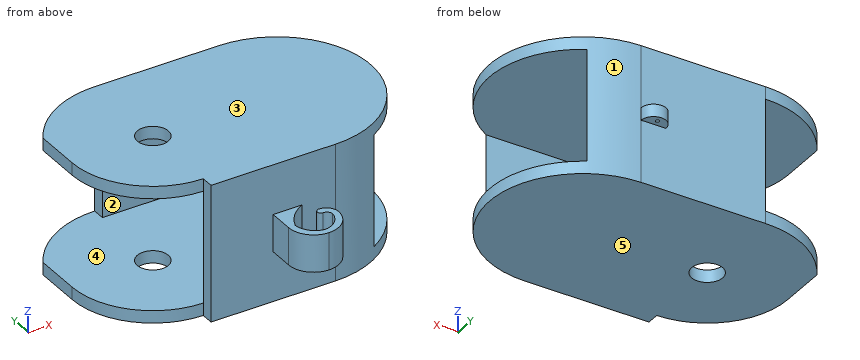
from build123d import *

# Parameters (mm, degrees)
SKETCH1_W           = 31.75
SKETCH1_H           = 19.05
BOSS_EXTRUDE1_DEPTH = 19.05
SKETCH2_R           = 1.5875
CUT_EXTRUDE2_DEPTH  = 19.05
SKETCH3_W           = 31.75
SKETCH3_H           = 2.54
SKETCH3_W_2         = 9.525
SKETCH3_H_2         = 11.43
CUT_EXTRUDE3_DEPTH  = 19.05
SKETCH4_W           = 11.43
SKETCH4_H           = 16.51
CUT_EXTRUDE4_DEPTH  = 50.8
CUT_EXTRUDE5_DEPTH  = 19.05
SKETCH6_W           = 5.08
SKETCH6_H           = 3.81
BOSS_EXTRUDE2_DEPTH = 7.62
CUT_EXTRUDE6_DEPTH  = 19.05
SKETCH8_W           = 2.54
SKETCH8_H           = 1.27
BOSS_EXTRUDE3_DEPTH = 1.27
SKETCH9_R           = 0.1905
CUT_EXTRUDE7_DEPTH  = 19.05


with BuildPart() as part:
    # Sketch1 → Boss-Extrude1 (new body)
    with BuildSketch(Plane(origin=(0, 0, 0), x_dir=(1, 0, 0), z_dir=(0, 1, 0))):
        Rectangle(SKETCH1_W, SKETCH1_H)
    extrude(amount=BOSS_EXTRUDE1_DEPTH)

    # Sketch2 → Cut-Extrude2 (cut)
    with BuildSketch(Plane.XY.offset(9.525)):
        with Locations((-6.35, 9.525)):
            Circle(SKETCH2_R)
        with BuildLine():
            ThreePointArc((-6.35, 19.05), (-15.875, 9.525), (-6.35, 0))
            ThreePointArc((-6.35, 0), (-27.315146333, 9.525), (-6.35, 19.05))
        make_face()
        with BuildLine():
            ThreePointArc((6.35, 0), (15.875, 9.525), (6.35, 19.05))
            ThreePointArc((6.35, 19.05), (24.948138119, 9.525), (6.35, 0))
        make_face()
    extrude(amount=-CUT_EXTRUDE2_DEPTH, mode=Mode.SUBTRACT)

    # Sketch3 → Cut-Extrude3 (cut)
    with BuildSketch(Plane(origin=(0, 19.05, 0), x_dir=(1, 0, 0), z_dir=(0, 1, 0))):
        with Locations((0, 8.255)):
            Rectangle(SKETCH3_W, SKETCH3_H)
        with Locations((0, -8.255)):
            Rectangle(SKETCH3_W, SKETCH3_H)
        with Locations((-11.1125, 0)):
            Rectangle(SKETCH3_W_2, SKETCH3_H_2)
    extrude(amount=-CUT_EXTRUDE3_DEPTH, mode=Mode.SUBTRACT)

    # Sketch4 → Cut-Extrude4 (cut)
    with BuildSketch(Plane(origin=(-15.875, 0, 0), x_dir=(0, 0, -1), z_dir=(1, 0, 0))):
        with Locations((0, 9.525)):
            Rectangle(SKETCH4_W, SKETCH4_H)
    extrude(amount=CUT_EXTRUDE4_DEPTH, mode=Mode.SUBTRACT)

    # Sketch5 → Cut-Extrude5 (cut)
    with BuildSketch(Plane.XY.offset(9.525)):
        with BuildLine():
            Line((-14.605, 17.4863926), (-18.31070608, 1.27))
            Line((-18.31070608, 1.27), (-18.31070608, 0))
            Line((-18.31070608, 0), (-6.35, 0))
            Line((-6.35, 0), (-6.35, 1.27))
            ThreePointArc((-6.35, 1.27), (-12.187166479, 3.687833521), (-14.605, 9.525))
            Line((-14.605, 9.525), (-14.605, 17.4863926))
        make_face()
    extrude(amount=-CUT_EXTRUDE5_DEPTH, mode=Mode.SUBTRACT)

    # Sketch6 → Boss-Extrude2 (add)
    with BuildSketch(Plane(origin=(0, 0, 0), x_dir=(1, 0, 0), z_dir=(0, 1, 0))):
        with Locations((2.54, 0)):
            Rectangle(SKETCH6_W, SKETCH6_H)
    extrude(amount=-BOSS_EXTRUDE2_DEPTH)

    # Sketch7 → Cut-Extrude6 (cut)
    with BuildSketch(Plane.XY.offset(9.525)):
        with BuildLine():
            Line((0, -2.54), (0, 0))
            ThreePointArc((0, 0), (2.54, -9.543763037), (5.08, 0))
            Line((5.08, 0), (2.940211157, 0))
            ThreePointArc((2.940211157, 0), (1.549192819, -1.039121584), (0.676226805, -2.54))
            ThreePointArc((0.676226805, -2.54), (1.276666453, -3.82212392), (2.54, -4.461152767))
            ThreePointArc((2.54, -4.461152767), (3.830489938, -3.856329433), (4.454963278, -2.575232796))
            ThreePointArc((4.454963278, -2.575232796), (4.237571766, -2.189951454), (3.823346179, -2.034651919))
            ThreePointArc((3.823346179, -2.034651919), (3.463036915, -1.694231845), (3.803456989, -1.333922582))
            ThreePointArc((3.803456989, -1.333922582), (4.691515307, -1.672580577), (5.08, -2.54))
            ThreePointArc((5.08, -2.54), (4.336051224, -4.336051224), (2.54, -5.08))
            ThreePointArc((2.54, -5.08), (0.743948776, -4.336051224), (0, -2.54))
        make_face()
    extrude(amount=-CUT_EXTRUDE6_DEPTH, mode=Mode.SUBTRACT)

    # Sketch8 → Boss-Extrude3 (add)
    with BuildSketch(Plane(origin=(0, 19.05, 0), x_dir=(1, 0, 0), z_dir=(0, 1, 0))):
        with Locations((5.08, 0)):
            Rectangle(SKETCH8_W, SKETCH8_H)
    extrude(amount=BOSS_EXTRUDE3_DEPTH)

    # Sketch9 → Cut-Extrude7 (cut)
    with BuildSketch(Plane.XY.offset(9.525)):
        with Locations((5.08, 19.685)):
            Circle(SKETCH9_R)
        with BuildLine():
            ThreePointArc((3.81, 19.05), (5.08, 20.32), (6.35, 19.05))
            ThreePointArc((6.35, 19.05), (5.08, 21.265981124), (3.81, 19.05))
        make_face()
    extrude(amount=-CUT_EXTRUDE7_DEPTH, mode=Mode.SUBTRACT)


solid = part.part
Could you check a few things on this model? Use its own coordinates, in mm. Face numbers are marked on the shaded views. A direction names the side the tool comes from. Give positions to 0.01 mm unless a question says otherwise; leave off trailing zeros. Order: outer loops, then holes, each group sorted by start corner. A loop starts at its lowest first (then second) coordinate and runs counter-clockwise, first axis right, second up. Notation, with made-up numbers: (-11, -40) - (31, -40) arc R25 cw to (31, -23) - close; hole circle Ø10 at (-12, 32.25). An arc over 180 degrees is marked (long way). One line per question, with ' | ' between items. Start each with the question number.
Item 1: For the marked faces 1 and 2, which set-ups out of +Z, -Z, +X, -X, +Y, -Y let a thin tool reach every point of the face, with its end or its side?
Item 2: I'm going to push flat-ended pins straight in: pin 1 Ø1 at (y, z) = (0.5, -2.5) entering from -X; pin 2 Ø5 at (y, z) = (0.5, -4) entering from -X; pin 3 Ø1.3 at (y, z) = (-1.5, 0.5) entering from -X. Where does each tip first touch, or does it pass through?
Item 3: I want a section at B-B on y = 6.25. Write out the boundary of the cut face in (x, z) (3 decimals).
Item 4: I want a section at D-D on z = -0.25. Give the number of separate pieces and of enclosed holes in the cut face, then the cut area to 3 significant figures.
Item 5: I need wall thicknesses on probe 1 along Z at (x, y) = (9, 15) (3 decimals); probe 2 along Y at (x, z) = (-3, -2.5). Which ranges of each line are inside material? Lowest first, please. Write a range as [from, to].
Item 6: I want a section at C-C on x = 1.5. Write out the boundary of the cut face in (y, z) (3 decimals), then the cut area to 3 significant figures.
Item 7: I want a section at A-A on z = 4. Write out the boundary of the cut face in (x, y) (3 decimals), then the cut area to 3 significant figures.
Item 8: Thinking about a two-plate mould opening in Z: for the marked faces 3, 4 and 5, which applies, pulls with the +Z half, pulls with the -Z half, needs draft (parallel to the pull), parting line crosses it, or undercut?
Verdict:
1) face 1: +Z, -Z, +X | face 2: +X, -X
2) pin 1: x = -6.35 | pin 2: x = -10.38 | pin 3: x = 0
3) outline: (-13.928, -6.985) - (15.294, -6.985) - (15.294, -5.715) - (-13.928, -5.715) - close; (-13.928, 5.715) - (15.294, 5.715) - (15.294, 6.985) - (-13.928, 6.985) - close
4) separate pieces: 2 | enclosed holes: 1 | area: 52.5 mm^2
5) probe 1: [-6.985, -5.715], [5.715, 6.985] | probe 2: [0, 1.27], [17.78, 19.05]
6) outline: (-4.857, -1.905) - (-4.023, -1.905) - (-4.023, 1.905) - (-4.857, 1.905) - close; (-1.095, -1.905) - (0, -1.905) - (0, -6.985) - (19.05, -6.985) - (19.05, 6.985) - (0, 6.985) - (0, 1.905) - (-1.095, 1.905) - close; hole (1.27, -5.715) - (17.78, -5.715) - (17.78, 5.715) - (1.27, 5.715) - close | area: 84.8 mm^2
7) outline: (-6.35, 0) - (6.35, 0) arc R9.525 ccw to (11.102, 1.27) - (-6.35, 1.27) - close; (-6.35, 17.78) - (11.102, 17.78) arc R9.525 ccw to (6.35, 19.05) - (-6.35, 19.05) - close | area: 40.4 mm^2
8) face 3: pulls with the +Z half | face 4: undercut | face 5: pulls with the -Z half
